Here's the drawing with two shaded views (mm, measured from the low corner). I have some questions. A direction names the side the tool comes from. Round coordinates to 2 decimals unless told otherwise and drop trailing zeros. Order: outer loops, then holes, each group sorted by start corner. A loop starts at its lowest first (then second) coordinate and runs counter-clockwise, first axis right, second up.
Q1. If we section it at C-C (z = 30): Please give me the cut outline in (x, y) (1 decimal).
Q2. Will these pins go through, and if not, where does the flat tip stop? P1, Ø10.5, axis at x = 33, z = 29, coming from the -Y side; P2, Ø2, axis at y = 4.5, z = 26, coming from the +X side; P3, Ø2, axis at x = 15.5, y = 5, coming from the -Z side; P4, Ø1.3, axis at y = 5, z = 20, coming from the -X side (1 decimal).
Q3. If we section it at B-B (z = 36.5): Please give me the cut outline in (x, y) (1 decimal), plus the area to 3 significant figures.
Q4. For the marked faces 1, 2 and 3, which set-ups out of +Z, -Z, +X, -X, +Y, -Y let a thin tool reach every point of the face, with its end or its side?
Q5. If I drill on line 1 (Y direction, x = 36, z = 3); line 2 (Y direction, x = 13, z = 32); line 3 (X direction, y = 3.5, z = 14) (1 decimal), over which ranges is the centre line in solid material (lowest first)?
Q6. If we section it at D-D (x = 30.5): Please give me the cut outline in (y, z) (1 decimal).
Q7. If we section it at A-A (x = 8): Please give me the cut outline in (y, z) (1 decimal).
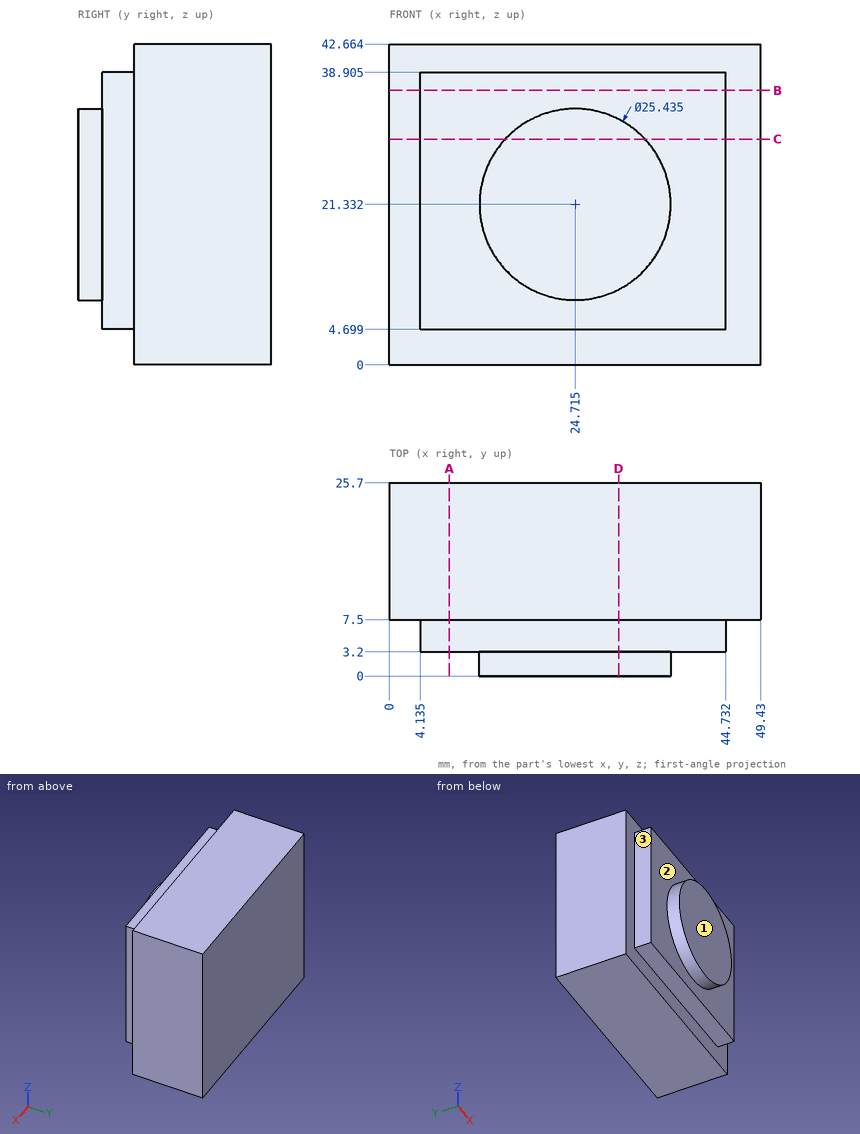
Solution:
1. outline: (0, 7.5) - (4.1, 7.5) - (4.1, 3.2) - (15.4, 3.2) - (15.4, 0) - (34, 0) - (34, 3.2) - (44.7, 3.2) - (44.7, 7.5) - (49.4, 7.5) - (49.4, 25.7) - (0, 25.7) - close
2. P1: stops at y = 0
2. P2: stops at x = 44.73
2. P3: stops at z = 4.7
2. P4: stops at x = 4.1
3. outline: (0, 7.5) - (4.1, 7.5) - (4.1, 3.2) - (44.7, 3.2) - (44.7, 7.5) - (49.4, 7.5) - (49.4, 25.7) - (0, 25.7) - close
3. area: 1,070 mm2
4. face 1: +Z, -Z, +X, -X, -Y
4. face 2: -Y
4. face 3: +Z, -Z, -X, -Y
5. line 1: y = 7.5 to 25.7
5. line 2: y = 3.2 to 25.7
5. line 3: x = 4.1 to 44.7
6. outline: (0, 10) - (3.2, 10) - (3.2, 4.7) - (7.5, 4.7) - (7.5, 0) - (25.7, 0) - (25.7, 42.7) - (7.5, 42.7) - (7.5, 38.9) - (3.2, 38.9) - (3.2, 32.7) - (0, 32.7) - close
7. outline: (3.2, 4.7) - (7.5, 4.7) - (7.5, 0) - (25.7, 0) - (25.7, 42.7) - (7.5, 42.7) - (7.5, 38.9) - (3.2, 38.9) - close
